```python
from build123d import *

# Parameters (mm, degrees)
SKETCH1_W           = 3.175
SKETCH1_H           = 3.175
BOSS_EXTRUDE1_DEPTH = 120.65
SKETCH2_OUTSIDE_W   = 29.322
SKETCH2_OUTSIDE_H   = 29.322
SKETCH2_OUTSIDE_R   = 2.032
CUT_EXTRUDE1_DEPTH  = 121.65


with BuildPart() as part:
    # Sketch1 → Boss-Extrude1 (new body)
    with BuildSketch(Plane.XY):
        Rectangle(SKETCH1_W, SKETCH1_H)
    extrude(amount=BOSS_EXTRUDE1_DEPTH)

    # Sketch2 outside → Cut-Extrude1 (cut, through all)
    with BuildSketch(Plane(origin=(0, 0, 0), x_dir=(-1, 0, 0), z_dir=(0, 0, -1))):
        Rectangle(SKETCH2_OUTSIDE_W, SKETCH2_OUTSIDE_H)
        Circle(SKETCH2_OUTSIDE_R, mode=Mode.SUBTRACT)
    extrude(amount=-CUT_EXTRUDE1_DEPTH, mode=Mode.SUBTRACT)

    # Sketch3 → Cut-Revolve1 (revolve, cut)
    with BuildSketch(Plane(origin=(0, 0, 0), x_dir=(1, 0, 0), z_dir=(0, 1, 0))):
        with BuildLine():
            Line((-5.053685963, -4.40273269), (-5.053685963, 5.740530545))
            Line((-5.053685963, 5.740530545), (0, 5.740530545))
            Line((0, 5.740530545), (0, 0.160877736))
            ThreePointArc((0, 0.160877736), (-3.404639553, -1.148866368), (-5.053685963, -4.40273269))
        make_face()
    revolve(axis=Axis((0, 0, 120.65), (0, 0, -1)), mode=Mode.SUBTRACT)

    # Mirror1: part across plane


with BuildPart() as part_1:
    add(part.part)
    add(part.part.mirror(Plane(origin=(0, 0, 120.65), x_dir=(1, 0, 0), z_dir=(0, 0, -1))))


solid = part_1.part
```
For this review, take the finished solid that the model builds, in its own axes (mm). Coordinates: 2 decimals unless noted, no trailing zeros. Write each loop counter-clockwise with the first axis right and the second up, starting at its lowest first coordinate (ties: lowest second). Pieces come first, ordered by that corner, then holes. Notation, with made-up numbers: (45.5, 68.5) -> (51.5, 68.5) arc R23 cw to (51.5, 104.5) -> close; hole circle Ø2 at (-5, 48). An arc over 180 degrees is marked (long way). Put each result on its own line as item: value.
Q1. Take a section at A-A, the plane z = 127. State the section outline as (x, y) points, then the cut area to 3 significant figures.
From the geometry:
outline: (-1.59, -1.27) arc R2.03 ccw to (-1.27, -1.59) -> (1.27, -1.59) arc R2.03 ccw to (1.59, -1.27) -> (1.59, 1.27) arc R2.03 ccw to (1.27, 1.59) -> (-1.27, 1.59) arc R2.03 ccw to (-1.59, 1.27) -> close
area: 9.89 mm2
Q2. Wall thickness on L1, parallel to Z at x = 1.35, y = -0.15; L2, parallel to Y at x = -1.35, z = 68; L3, parallel to Z at x = 1.3, y = 0.8: over which ranges is each line inside the solid? List them lowest first.
From the geometry:
L1: z = 0.02 to 241.28
L2: y = -1.52 to 1.52
L3: z = 0.07 to 241.23
Q3. Clearance check with a flat-ended pin moving along its axis: pin 1 Ø1.5 at (x, y) = (-0.5, -0.5) entering from -Z. State where the tip first meets the part, or that it passes through.
From the geometry:
pin 1: stops at z = 0
